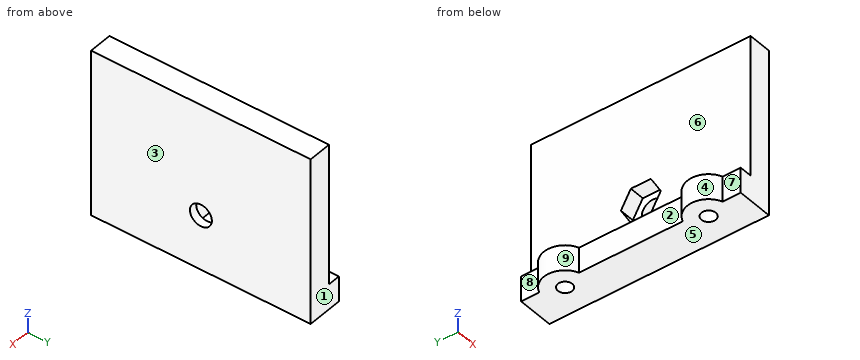
```python
from build123d import *

# Parameters (mm, degrees)
SKETCH1_W           = 39.5
SKETCH1_H           = 52
SKETCH1_R           = 2.6
BOSS_EXTRUDE1_DEPTH = 5.5
CUT_EXTRUDE1_DEPTH  = 3.6
SKETCH3_W           = 8.5
SKETCH3_H           = 52
BOSS_EXTRUDE2_DEPTH = 6
SKETCH4_R           = 5.05
SKETCH4_R_2         = 1.7
BOSS_EXTRUDE3_DEPTH = 6
SKETCH5_R           = 5.05
SKETCH5_R_2         = 1.7
BOSS_EXTRUDE4_DEPTH = 6
SKETCH6_R           = 1.7
CUT_EXTRUDE2_DEPTH  = 6


with BuildPart() as part:
    # Sketch1 → Boss-Extrude1 (new body)
    with BuildSketch(Plane(origin=(330.5, 0, 0), x_dir=(0, 0, -1), z_dir=(1, 0, 0))):
        with Locations((-306.75, 300)):
            Rectangle(SKETCH1_W, SKETCH1_H)
        with Locations((-300, 300)):
            Circle(SKETCH1_R, mode=Mode.SUBTRACT)
    extrude(amount=BOSS_EXTRUDE1_DEPTH)

    # Sketch2 → Cut-Extrude1 (cut)
    with BuildSketch(Plane(origin=(330.5, 0, 0), x_dir=(0, 0, -1), z_dir=(1, 0, 0))):
        Polygon((-304.1, 302.367136104), (-300, 304.734272207), (-295.9, 302.367136104), (-295.9, 297.632863896), (-300, 295.265727793), (-304.1, 297.632863896), align=None)
    extrude(amount=CUT_EXTRUDE1_DEPTH, mode=Mode.SUBTRACT)

    # Sketch3 → Boss-Extrude2 (add)
    with BuildSketch(Plane.XY.offset(287)):
        with Locations((331.75, 300)):
            Rectangle(SKETCH3_W, SKETCH3_H)
    extrude(amount=BOSS_EXTRUDE2_DEPTH)

    # Sketch4 → Boss-Extrude3 (add)
    with BuildSketch(Plane.XY.offset(287)):
        with Locations((329.3, 283)):
            Circle(SKETCH4_R)
        with Locations((329.3, 283)):
            Circle(SKETCH4_R_2, mode=Mode.SUBTRACT)
    extrude(amount=BOSS_EXTRUDE3_DEPTH)

    # Sketch5 → Boss-Extrude4 (add)
    with BuildSketch(Plane.XY.offset(287)):
        with Locations((329.3, 317)):
            Circle(SKETCH5_R)
        with Locations((329.3, 317)):
            Circle(SKETCH5_R_2, mode=Mode.SUBTRACT)
    extrude(amount=BOSS_EXTRUDE4_DEPTH)

    # Sketch6 → Cut-Extrude2 (cut)
    with BuildSketch(Plane.XY.offset(287)):
        with Locations(Location((329.3, 283, 0), (0, 0, 314.900872156))):
            Circle(SKETCH6_R)
        with Locations(Location((329.3, 317, 0), (0, 0, 314.900872156))):
            Circle(SKETCH6_R)
    extrude(amount=CUT_EXTRUDE2_DEPTH, mode=Mode.SUBTRACT)


solid = part.part
```
Can you work these out from the model? Positions are in its coordinate system, mm. Face numbers are marked on the shaded views. A direction names the side the tool comes from. Give positions to 0.01 mm unless a question says otherwise; leave off trailing zeros. Loops run counter-clockwise (first coordinate to the right, second up) from the corner with the lowest first, then second, coordinate; pieces in that order, holes last. Notation, with made-up numbers: M 81,8.25 L 97,8.25 A25 ccw 97,32.25 Z; hole C -16.5,19 d6. An arc over 180 degrees is marked long. Answer in a Markdown table with one row per item.
1. Which directions (+Z, -Z, +X, -X, +Y, -Y) give clear straight access to the entire face, cutting with the end or side of a thin tool? Please do the marked faces 5, 6, 7, 8 and 9.
Taken from the geometry:
| item | result |
|---|---|
| face 5 | -Z, +X, -X, +Y, -Y |
| face 6 | +Z, -X, +Y, -Y |
| face 7 | +Z, -Z, -X, -Y |
| face 8 | +Z, -Z, -X, +Y |
| face 9 | +Z, -Z, -X |
2. Suppose I cut it at A-A on y = 317. Write out the boundary of the cut face in (x, z), plus the area to 3 significant figures.
Taken from the geometry:
| item | result |
|---|---|
| outline | M 324.25,287 L 327.6,287 L 327.6,293 L 324.25,293 Z; M 330.5,293 L 331,293 L 331,287 L 336,287 L 336,326.5 L 330.5,326.5 Z |
| area | 234 mm² |
3. For pin 1 Ø17 at (y, z) = (303.5, 306) entering from -X; pin 2 Ø1 at (x, z) = (328, 294) entering from -Y; pin 3 Ø2.5 at (x, y) = (329.3, 317) entering from +Z; pin 4 Ø8 at (y, z) = (300.5, 295.5) entering from -X, each with a flat end and sliding along its axis, tell me the tip position at first contact or that it passes through.
Taken from the geometry:
| item | result |
|---|---|
| pin 1 | stops at x = 330.5 |
| pin 2 | passes through |
| pin 3 | stops at z = 326.5 |
| pin 4 | stops at x = 327.5 |
4. If I drill on line 1 along Y through (x, z) = (329.3, 289.9); line 2 along Z through (x, y) = (335, 300); line 3 along Y through (x, z) = (335, 300), over which ranges is the centre line in solid material (lowest first)?
Taken from the geometry:
| item | result |
|---|---|
| line 1 | y = 274 to 281.3, 284.7 to 315.3, 318.7 to 326 |
| line 2 | z = 287 to 297.4, 302.6 to 326.5 |
| line 3 | y = 274 to 297.4, 302.6 to 326 |
5. Suppose I cut it at C-C on z = 301.5. Write out the boundary of the cut face in (x, y).
Taken from the geometry:
| item | result |
|---|---|
| outline | M 330.5,274 L 336,274 L 336,297.88 L 334.1,297.88 L 334.1,296.13 L 330.5,296.13 Z; M 330.5,303.87 L 334.1,303.87 L 334.1,302.12 L 336,302.12 L 336,326 L 330.5,326 Z |
6. Suppose I cut it at D-D on y = 299. Write out the boundary of the cut face in (x, z).
Taken from the geometry:
| item | result |
|---|---|
| outline | M 327.5,287 L 336,287 L 336,297.6 L 334.1,297.6 L 334.1,295.9 L 330.5,295.9 L 330.5,293 L 327.5,293 Z; M 330.5,304.1 L 334.1,304.1 L 334.1,302.4 L 336,302.4 L 336,326.5 L 330.5,326.5 Z |
7. Thinking about a two-plate mould opening in Y: for the marked faces 1, 2, 3 and 4, which applies, released by +Y, released by -Y, zero draft, split by the parting line, or undercut?
Taken from the geometry:
| item | result |
|---|---|
| face 1 | released by +Y |
| face 2 | undercut |
| face 3 | zero draft |
| face 4 | undercut |
8. Suppose I cut it at B-B on x = 328.5. Write out the boundary of the cut face in (y, z), plus the area to 3 significant figures.
Taken from the geometry:
| item | result |
|---|---|
| outline | M 274,287 L 281.5,287 L 281.5,293 L 274,293 Z; M 284.5,287 L 315.5,287 L 315.5,293 L 284.5,293 Z; M 318.5,287 L 326,287 L 326,293 L 318.5,293 Z |
| area | 276 mm² |
